The model under review builds one solid part; all positions refer to its coordinate system, in mm. Face numbers are marked on the shaded views. A direction names the side the tool comes from. Round coordinates to 2 decimals unless told otherwise and drop trailing zeros. Write each loop counter-clockwise with the first axis right and the second up, starting at its lowest first coordinate (ties: lowest second). Pieces come first, ordered by that corner, then holes. Notation, with made-up numbers: (-37, -17.75) - (-22, -17.75) arc R16 cw to (-22, 6.25) - close; hole circle Ø5 at (11.25, -2). An arc over 180 degrees is marked (long way). Return JSON: item names as keys, results as strings.
from build123d import *

# Parameters (mm, degrees)
F1_DEPTH      = 75
F3_DEPTH      = 30
F3_DEPTH_BACK = 90
F4_W          = 68.7531680209
F4_H          = 14.4708263688
F5_DEPTH      = 25
F5_DEPTH_BACK = 10


with BuildPart() as f1:
    # F0 (on Front) → F1 (new body)
    with BuildSketch(Plane.XZ):
        with BuildLine():
            Line((35.7055822906, 78.3045381219), (-54.2122411279, -6.6178094916))
            ThreePointArc((-54.2122411279, -6.6178094916), (-54.5952252844, -6.8622663067), (-55.0413462098, -6.9483599686))
            ThreePointArc((-55.0413462098, -6.9483599686), (-65.454548531, -1.0579541733), (-65.7249668893, 10.9027538713))
            ThreePointArc((-65.7249668893, 10.9027538713), (-65.7514161094, 12.0978334092), (-66.7910191515, 12.6878674574))
            Line((-66.7910191515, 12.6878674574), (-69.3984164298, 12.6878674574))
            ThreePointArc((-69.3984164298, 12.6878674574), (-69.6958292502, 12.6199768131), (-69.9343224371, 12.4297545087))
            Line((-69.9343224371, 12.4297545087), (-71.4332162747, 10.549801355))
            ThreePointArc((-71.4332162747, 10.549801355), (-72.983516127, 0.1409632474), (-67.6478594542, -8.9297648519))
            ThreePointArc((-67.6478594542, -8.9297648519), (-65.2384193211, -13.915925777), (-67.3571118078, -19.0324035373))
            Line((-67.3571118078, -19.0324035373), (-109.6802590447, -59.0042454993))
            ThreePointArc((-109.6802590447, -59.0042454993), (-109.3628044531, -67.2017482376), (-102.1890001615, -71.1812407363))
            Line((-102.1890001615, -71.1812407363), (-53.1669473059, -71.1812407356))
            ThreePointArc((-53.1669473059, -71.1812407356), (-51.1816807122, -70.9332267187), (-49.3184445074, -70.2044295966))
            Line((-49.3184445074, -70.2044295966), (8.606172505, -38.7753114248))
            ThreePointArc((8.606172505, -38.7753114248), (12.2860183049, -37.8002629481), (16.0033975224, -38.6206752819))
            Line((16.0033975224, -38.6206752819), (54.5573614144, -57.4984885011))
            ThreePointArc((54.5573614144, -57.4984885011), (54.7053822121, -57.5790589788), (54.8459093451, -57.6720852296))
            Line((54.8459093451, -57.6720852296), (69.2774157369, -68.1477812421))
            ThreePointArc((69.2774157369, -68.1477812421), (72.0938830707, -69.5760831015), (75.2153037267, -70.0549019945))
            Line((75.2153037267, -70.0549019945), (78.6547126816, -70.03306521))
            Line((78.6547126816, -70.03306521), (88.6365619759, -69.9696905154))
            ThreePointArc((88.6365619759, -69.9696905154), (99.1815473838, -65.542870992), (103.5413289953, -54.9699928292))
            Line((103.5413289953, -54.9699928292), (103.5413289953, -54.1190856195))
            ThreePointArc((103.5413289953, -54.1190856195), (101.8167785406, -47.1360748524), (97.0396704124, -41.7587380046))
            Line((97.0396704124, -41.7587380046), (74.9481714859, -26.5697557736))
            ThreePointArc((74.9481714859, -26.5697557736), (73.5068370972, -26.2547430485), (72.2561461348, -27.0373348667))
            Line((72.2561461348, -27.0373348667), (70.7882150116, -29.0739654592))
            ThreePointArc((70.7882150116, -29.0739654592), (69.371825982, -34.9724326755), (72.5013272631, -40.1689983795))
            Line((72.5013272631, -40.1689983795), (90.4884265587, -53.557894228))
            ThreePointArc((90.4884265587, -53.557894228), (91.510056882, -56.0523850299), (89.7824317217, -58.1215694547))
            ThreePointArc((89.7824317217, -58.1215694547), (83.3025731901, -59.9380088951), (76.7556883533, -58.3803446938))
            Line((76.7556883533, -58.3803446938), (15.9965307599, -26.203911059))
            ThreePointArc((15.9965307599, -26.203911059), (12.1791348203, -25.2657414738), (8.3714169644, -26.2424495468))
            Line((8.3714169644, -26.2424495468), (-46.4835128256, -56.0059967154))
            ThreePointArc((-46.4835128256, -56.0059967154), (-65.7620061585, -51.6527529228), (-63.9911285633, -31.9683675057))
            Line((-63.9911285633, -31.9683675057), (43.2786946767, 70.3661996968))
            Line((43.2786946767, 70.3661996968), (35.7055822906, 78.3045381219))
        make_face()
    extrude(amount=F1_DEPTH)

    # F2 (on face) → F3 (cut, two sides)
    with BuildSketch(Plane(origin=(-22.2549429173, 0, 23.5640686305), x_dir=(0.7270133187, 0, 0.686623357), z_dir=(-0.686623357, 0, 0.7270133187))) as f3_sk:
        Polygon((-43.9569639067, -24.1313080694), (-143.9990401268, -21.0843849927), (-143.4555607145, -53.2556629783), (-43.9569639067, -50.5866528074), align=None)
        with BuildLine():
            Line((-18.389185364, -24.9100109652), (-43.9569639067, -24.1313080694))
            Line((-43.9569639067, -24.1313080694), (-43.9569639067, -50.5866528074))
            Line((-43.9569639067, -50.5866528074), (-18.4254588112, -49.9017803673))
            ThreePointArc((-18.4254588112, -49.9017803673), (-11.5283625374, -46.8809946351), (-8.6936083649, -39.905376223))
            Line((-8.6936083649, -39.905376223), (-8.6936083649, -34.905376223))
            ThreePointArc((-8.6936083649, -34.905376223), (-11.5157176577, -27.9427700303), (-18.389185364, -24.9100109652))
        make_face()
    extrude(amount=F3_DEPTH, mode=Mode.SUBTRACT)
    extrude(f3_sk.sketch, amount=-F3_DEPTH_BACK, mode=Mode.SUBTRACT)

    # F4 (on face) → F5 (cut, two sides)
    with BuildSketch(Plane(origin=(-7.3339171449, 0, -13.8487264512), x_dir=(0.8837288425, 0, -0.4679992873), z_dir=(0.4679992873, 0, 0.8837288425))) as f5_sk:
        with Locations((60.7765913236, -37.6946638618)):
            Rectangle(F4_W, F4_H)
        with BuildLine():
            ThreePointArc((11.2418346107, -39.9300770462), (12.7063007048, -43.4656109521), (16.2418346107, -44.9300770462))
            Line((16.2418346107, -44.9300770462), (26.4000073131, -44.9300770462))
            Line((26.4000073131, -44.9300770462), (26.4000073131, -30.4592506774))
            Line((26.4000073131, -30.4592506774), (16.2418346107, -30.4592506774))
            ThreePointArc((16.2418346107, -30.4592506774), (12.7063007048, -31.9237167714), (11.2418346107, -35.4592506774))
            Line((11.2418346107, -35.4592506774), (11.2418346107, -39.9300770462))
        make_face()
        with BuildLine():
            Line((95.153175334, -30.4592506774), (95.153175334, -44.9300770462))
            Line((95.153175334, -44.9300770462), (131.284661945, -44.9300770462))
            ThreePointArc((131.284661945, -44.9300770462), (134.8201958509, -43.4656109521), (136.284661945, -39.9300770462))
            Line((136.284661945, -39.9300770462), (136.284661945, -35.4592506774))
            ThreePointArc((136.284661945, -35.4592506774), (134.8201958509, -31.9237167714), (131.284661945, -30.4592506774))
            Line((131.284661945, -30.4592506774), (95.153175334, -30.4592506774))
        make_face()
    extrude(amount=-F5_DEPTH, mode=Mode.SUBTRACT)
    extrude(f5_sk.sketch, amount=F5_DEPTH_BACK, mode=Mode.SUBTRACT)


solid = f1.part
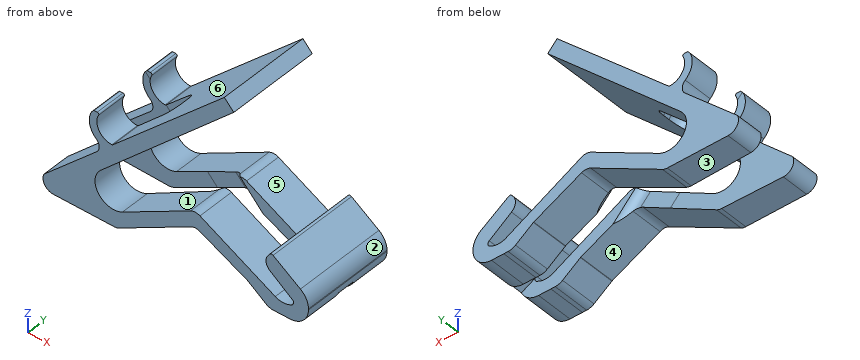
(1) Wall thickness on line 1 (X direction, y = -15.5, z = -50.5); line 2 (X direction, y = -4, z = 8); line 3 (Z direction, x = 43, y = -63.5): over which ranges is each line inside the solid? List them lowest first.
Filled in:
{"line 1": "x = -100.68 to -66.52, -36.34 to -13, 40.26 to 61.88, 86.38 to 103.1", "line 2": "x = -72.51 to -66.84, -38.73 to -22.1", "line 3": "z = -51.84 to -40.5, 70.1 to 70.66"}
(2) Add section A-A (z = -3). Write out the cut boundary in (x, y), plus the area to 3 significant figures.
Filled in:
{"outline": "(-72.03, -75) - (-64.01, -75) - (-64.01, -50.71) - (-72.03, -50.87) - close; (-72.03, -23.81) - (-64.01, -23.99) - (-64.01, 0) - (-72.03, 0) - close; (-50.38, -75) - (-33.63, -75) - (-33.63, -50.12) - (-50.38, -50.45) - close; (-50.38, -24.29) - (-33.63, -24.66) - (-33.63, 0) - (-50.38, 0) - close", "area": "1,210 mm2"}
(3) For the marked faces 4, 5 and 6, list the 3-axis set-ups (+Z, -Z, +X, -X, +Y, -Y) from which the entire face can be reached by the end or side of a thin tool; tool diameter is ignored.
Filled in:
{"face 4": "-Z, +Y, -Y", "face 5": "+Y, -Y", "face 6": "+Z, +Y, -Y"}
(4) Clearance check with flat-ended pins moving along their axes: pin 1 Ø8 at (y, z) = (-7.5, 25.5) entering from +X; pin 2 Ø8 at (y, z) = (-20.5, -51) entering from -X; pin 3 Ø1 at (x, y) = (61, -28) entering from -Z. State where each tip first meets the part, or that it passes through.
Filled in:
{"pin 1": "stops at x = 0.44", "pin 2": "stops at x = -105.44", "pin 3": "stops at z = -62.5"}
(5) Add section C-C (z = 64). Write out the cut boundary in (x, y), plus the area to 3 significant figures.
Filled in:
{"outline": "(20.56, -75) - (36.61, -75) - (36.61, 0) - (20.56, 0) - close", "area": "1,200 mm2"}
(6) Mouldability with a two-part tool opening along Z and no side actions: class the marked faces 1, 2 and 3 as released by +Z, released by -Z, zero draft, split by the parting line, or undercut.
Filled in:
{"face 1": "undercut", "face 2": "released by +Z", "face 3": "released by -Z"}
(7) Add section B-B (x = 21.5). Give the number of separate pieces and of enclosed holes in the cut face, plus the area to 3 significant figures.
Filled in:
{"separate pieces": "3", "enclosed holes": "0", "area": "1,870 mm2"}
